For this review, take the finished solid that the model builds, in its own axes (mm). Face numbers are marked on the shaded views. A direction names the side the tool comes from. Round coordinates to 2 decimals unless told otherwise and drop trailing zeros. Write each loop counter-clockwise with the first axis right and the second up, starting at its lowest first coordinate (ties: lowest second). Pieces come first, ordered by that corner, then holes. Notation, with made-up numbers: M 33,-31.75 L 59,-31.75 A5 ccw 59,-22.75 Z; hole C 39,-28 d4. An arc over 180 degrees is marked long. One line per question, with ' | ' between items.
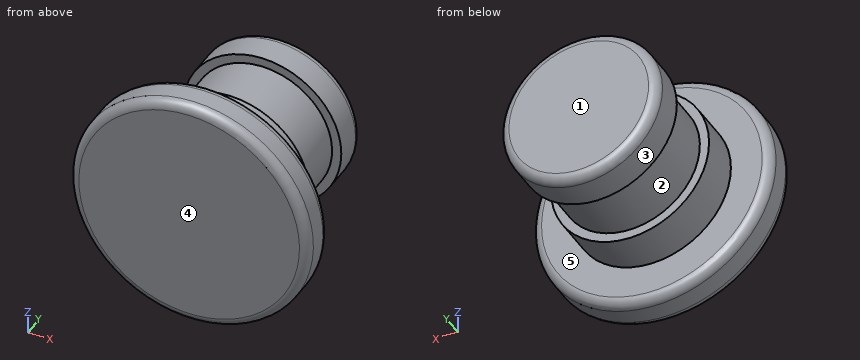
```python
from build123d import *

# Parameters (mm, degrees)
ESBO_O1_R                = 6.5
RESSALTO_EXTRUS_O1_DEPTH = 2
ESBO_O2_R                = 4.3
RESSALTO_EXTRUS_O2_DEPTH = 2.3
ESBO_O3_R                = 3.8
RESSALTO_EXTRUS_O3_DEPTH = 3.4
ESBO_O4_R                = 4.3
RESSALTO_EXTRUS_O4_DEPTH = 2
FILETE1_R                = 0.5


with BuildPart() as part:
    # Esboço1 → Ressalto-extrusão1 (new body)
    with BuildSketch(Plane(origin=(0, 0, 0), x_dir=(1, 0, 0), z_dir=(0, 1, 0))):
        with Locations(Location((0, 0, 0), (0, 0, 270))):
            Circle(ESBO_O1_R)
    extrude(amount=-RESSALTO_EXTRUS_O1_DEPTH)

    # Esboço2 → Ressalto-extrusão2 (add)
    with BuildSketch(Plane(origin=(0, 0, 0), x_dir=(1, 0, 0), z_dir=(0, 1, 0))):
        with Locations(Location((0, 0, 0), (0, 0, 270))):
            Circle(ESBO_O2_R)
    extrude(amount=RESSALTO_EXTRUS_O2_DEPTH)

    # Esboço3 → Ressalto-extrusão3 (add)
    with BuildSketch(Plane(origin=(0, 2.3, 0), x_dir=(1, 0, 0), z_dir=(0, 1, 0))):
        with Locations(Location((0, 0, 0), (0, 0, 270))):
            Circle(ESBO_O3_R)
    extrude(amount=RESSALTO_EXTRUS_O3_DEPTH)

    # Esboço4 → Ressalto-extrusão4 (add)
    with BuildSketch(Plane(origin=(0, 5.7, 0), x_dir=(1, 0, 0), z_dir=(0, 1, 0))):
        with Locations(Location((0, 0, 0), (0, 0, 270))):
            Circle(ESBO_O4_R)
    extrude(amount=RESSALTO_EXTRUS_O4_DEPTH)

    # Filete1
    filete1_edges = [part.edges().sort_by_distance(p)[0] for p in [
        (0, 7.7, -4.3),
        (0, 0, -6.5),
        (0, -2, -6.5),
    ]]
    fillet(filete1_edges, radius=FILETE1_R)


solid = part.part
```
Item 1: Take a section at D-D (y = 6.75). Write out the cut boundary in (x, z).
Results:
outline: C 0,0 d8.6
Item 2: Insertion check: pin 1 Ø1 at (x, y) = (3, 4.5) entering from -Z; pin 2 Ø1 at (y, z) = (4, 3.5) entering from +X; pin 3 Ø5 at (y, z) = (3, 4) entering from -X. Each pin has a flat end and moves straight along its axis. Give the tip position at first contact, or say it passes through.
Results:
pin 1: z = -2.86 | pin 2: x = 2.33 | pin 3: x = -3.99
Item 3: Mouldability with a two-part tool opening along Y and no side actions: class the marked faces 1, 2 and 3 as +Y half, -Y half, draft (parallel to the pull), parting line (faces both ways), or undercut.
Results:
face 1: +Y half | face 2: undercut | face 3: draft
Item 4: Take a section at C-C (y = 4.75). Write out the cut boundary in (x, z), then the cut area to 3 significant figures.
Results:
outline: C 0,0 d7.6 | area: 45.4 mm2
Item 5: Take a section at B-B (x = 0). Write out the cut boundary in (y, z), then the cut area to 3 significant figures.
Results:
outline: M -2,-6 A0.5 ccw -1.5,-6.5 L -0.5,-6.5 A0.5 ccw 0,-6 L 0,-4.3 L 2.3,-4.3 L 2.3,-3.8 L 5.7,-3.8 L 5.7,-4.3 L 7.2,-4.3 A0.5 ccw 7.7,-3.8 L 7.7,3.8 A0.5 ccw 7.2,4.3 L 5.7,4.3 L 5.7,3.8 L 2.3,3.8 L 2.3,4.3 L 0,4.3 L 0,6 A0.5 ccw -0.5,6.5 L -1.5,6.5 A0.5 ccw -2,6 Z | area: 88.5 mm2
Item 6: Take a section at A-A (z = 0). Write out the cut boundary in (x, y).
Results:
outline: M -6.5,-1.5 A0.5 ccw -6,-2 L 6,-2 A0.5 ccw 6.5,-1.5 L 6.5,-0.5 A0.5 ccw 6,0 L 4.3,0 L 4.3,2.3 L 3.8,2.3 L 3.8,5.7 L 4.3,5.7 L 4.3,7.2 A0.5 ccw 3.8,7.7 L -3.8,7.7 A0.5 ccw -4.3,7.2 L -4.3,5.7 L -3.8,5.7 L -3.8,2.3 L -4.3,2.3 L -4.3,0 L -6,0 A0.5 ccw -6.5,-0.5 Z
Item 7: Machinability: for the marked faces 4 and 5, which of the approach directions +Z, -Z, +X, -X, +Y, -Y give a long, thin tool a straight path to every point of the face, cutting with its end or side? Answer none if there is none.
Results:
face 4: +Z, -Z, +X, -X, -Y | face 5: +Y
Item 8: To check wall thickness, follow line 1 along Y through (x, z) = (5, -0.75); line 2 along Y through (x, z) = (-4, 1); line 3 along Z through (x, y) = (5.5, -0.75). State the ranges of each line that lie inside material, in increasing order. Write a range as from..to.
Results:
line 1: -2..0 | line 2: -2..2.3, 5.7..7.58 | line 3: -3.46..3.46
